```python
from build123d import *

# Parameters (mm, degrees)
SKETCH1_W                    = 39.4
SKETCH1_H                    = 49.4
BOSS_EXTRUDE1_DEPTH          = 1
SKETCH2_R                    = 7.25
CUT_EXTRUDE1_DEPTH           = 32.609808604
BOSS_EXTRUDE2_START          = -1
SKETCH3_R                    = 2.2
SKETCH3_R_2                  = 1
BOSS_EXTRUDE2_DEPTH          = 10.4
SKETCH4_W                    = 39.4
SKETCH4_H                    = 49.4
SKETCH4_W_2                  = 27.4
SKETCH4_H_2                  = 37.4
BOSS_EXTRUDE4_DEPTH          = 9.4
SKETCH5_W                    = 39.4
SKETCH5_H                    = 6
BOSS_EXTRUDE5_DEPTH          = 10
SKETCH6_R                    = 1.65
CUT_EXTRUDE3_DEPTH           = 57.961478211
SKETCH7_R                    = 2.25
CUT_EXTRUDE4_DEPTH           = 57.961478211
BOSS_EXTRUDE6_START          = -9.4
BOSS_EXTRUDE6_DEPTH          = 9.4
SKETCH9_R                    = 1.1
CUT_EXTRUDE5_DEPTH           = 8
CUT_EXTRUDE5_DRAFT           = -2
CUT_EXTRUDE5_PROFILE_2_DEPTH = 8
CUT_EXTRUDE5_PROFILE_2_DRAFT = -2
CUT_EXTRUDE5_PROFILE_3_DEPTH = 8
CUT_EXTRUDE5_PROFILE_3_DRAFT = -2
CUT_EXTRUDE5_PROFILE_4_DEPTH = 8
CUT_EXTRUDE5_PROFILE_4_DRAFT = -2
CHAMFER1_SIZE                = 5


with BuildPart() as part:
    # Sketch1 → Boss-Extrude1 (new body)
    with BuildSketch(Plane.XY):
        Rectangle(SKETCH1_W, SKETCH1_H)
    extrude(amount=BOSS_EXTRUDE1_DEPTH)

    # Sketch2 → Cut-Extrude1 (cut, through all)
    with BuildSketch(Plane.XY.offset(1)):
        Circle(SKETCH2_R)
    extrude(amount=-CUT_EXTRUDE1_DEPTH, mode=Mode.SUBTRACT)

    # Sketch3 → Boss-Extrude2 (add)
    # profile 1 of 4: a face of its own
    with BuildSketch(Plane.XY.offset(1).offset(BOSS_EXTRUDE2_START)):
        with Locations(Location((-10.5, 4.98, 0), (0, 0, 180))):
            Circle(SKETCH3_R)
        with Locations(Location((-10.5, 4.98, 0), (0, 0, 180))):
            Circle(SKETCH3_R_2, mode=Mode.SUBTRACT)
    # profile 2 of 4: a face of its own
    with BuildSketch(Plane.XY.offset(1).offset(BOSS_EXTRUDE2_START)):
        with Locations(Location((-10.5, -7.52, 0), (0, 0, 180))):
            Circle(SKETCH3_R)
        with Locations(Location((-10.5, -7.52, 0), (0, 0, 180))):
            Circle(SKETCH3_R_2, mode=Mode.SUBTRACT)
    # profile 3 of 4: a face of its own
    with BuildSketch(Plane.XY.offset(1).offset(BOSS_EXTRUDE2_START)):
        with Locations(Location((10.5, -7.52, 0), (0, 0, 180))):
            Circle(SKETCH3_R)
        with Locations(Location((10.5, -7.52, 0), (0, 0, 180))):
            Circle(SKETCH3_R_2, mode=Mode.SUBTRACT)
    # profile 4 of 4: a face of its own
    with BuildSketch(Plane.XY.offset(1).offset(BOSS_EXTRUDE2_START)):
        with Locations(Location((10.5, 4.98, 0), (0, 0, 180))):
            Circle(SKETCH3_R)
        with Locations(Location((10.5, 4.98, 0), (0, 0, 180))):
            Circle(SKETCH3_R_2, mode=Mode.SUBTRACT)
    extrude(amount=BOSS_EXTRUDE2_DEPTH)

    # Sketch4 → Boss-Extrude4 (add)
    with BuildSketch(Plane.XY.offset(1)):
        Rectangle(SKETCH4_W, SKETCH4_H)
        Rectangle(SKETCH4_W_2, SKETCH4_H_2, mode=Mode.SUBTRACT)
    extrude(amount=BOSS_EXTRUDE4_DEPTH)

    # Sketch5 → Boss-Extrude5 (add)
    with BuildSketch(Plane.XY.offset(10.4)):
        with Locations((0, 21.7)):
            Rectangle(SKETCH5_W, SKETCH5_H)
        with Locations((0, -21.7)):
            Rectangle(SKETCH5_W, SKETCH5_H)
    extrude(amount=BOSS_EXTRUDE5_DEPTH)

    # Sketch6 → Cut-Extrude3 (cut, through all)
    with BuildSketch(Plane(origin=(0, 24.7, 0), x_dir=(1, 0, 0), z_dir=(0, 1, 0))):
        with Locations(Location((-12.5, -12.4, 0), (0, 0, 180))):
            Circle(SKETCH6_R)
        with Locations(Location((12.5, -12.4, 0), (0, 0, 180))):
            Circle(SKETCH6_R)
    extrude(amount=-CUT_EXTRUDE3_DEPTH, mode=Mode.SUBTRACT)

    # Sketch7 → Cut-Extrude4 (cut, through all)
    with BuildSketch(Plane(origin=(0, 24.7, 0), x_dir=(1, 0, 0), z_dir=(0, 1, 0))):
        with Locations(Location((12.5, -12.4, 0), (0, 0, 180))):
            Circle(SKETCH7_R)
        with Locations(Location((-12.5, -12.4, 0), (0, 0, 180))):
            Circle(SKETCH7_R)
    extrude(amount=-CUT_EXTRUDE4_DEPTH, mode=Mode.SUBTRACT)

    # Sketch8 → Boss-Extrude6 (add)
    with BuildSketch(Plane.XY.offset(10.4).offset(BOSS_EXTRUDE6_START)):
        with BuildLine():
            Line((-10.5, 7.18), (-13.7, 7.18))
            Line((-13.7, 7.18), (-13.7, 2.78))
            Line((-13.7, 2.78), (-10.5, 2.78))
            ThreePointArc((-10.5, 2.78), (-8.3, 4.98), (-10.5, 7.18))
        make_face()
        with BuildLine():
            Line((-10.5, -5.32), (-13.7, -5.32))
            Line((-13.7, -5.32), (-13.7, -9.72))
            Line((-13.7, -9.72), (-10.5, -9.72))
            ThreePointArc((-10.5, -9.72), (-8.3, -7.52), (-10.5, -5.32))
        make_face()
        with BuildLine():
            Line((10.5, 7.18), (13.7, 7.18))
            Line((13.7, 7.18), (13.7, 2.78))
            Line((13.7, 2.78), (10.5, 2.78))
            ThreePointArc((10.5, 2.78), (8.3, 4.98), (10.5, 7.18))
        make_face()
        with BuildLine():
            Line((10.5, -5.32), (13.7, -5.32))
            Line((13.7, -5.32), (13.7, -9.72))
            Line((13.7, -9.72), (10.5, -9.72))
            ThreePointArc((10.5, -9.72), (8.3, -7.52), (10.5, -5.32))
        make_face()
    extrude(amount=BOSS_EXTRUDE6_DEPTH)


with BuildPart() as cut_extrude5_tool:
    # Sketch9 → Cut-Extrude5 (with draft: the straight prism first)
    with BuildSketch(Plane.XY.offset(10.4)):
        with Locations((-10.5, 4.98)):
            Circle(SKETCH9_R)
    extrude(amount=-CUT_EXTRUDE5_DEPTH)
    # Cut-Extrude5: the draft: its side faces are tilted about the plane it starts from
    cut_extrude5_sides = [cut_extrude5_tool.faces().sort_by_distance(p)[0] for p in [
        (-11.6, 4.98, 6.4),
    ]]
    draft(cut_extrude5_sides, Plane.XY.offset(10.4), CUT_EXTRUDE5_DRAFT)


with BuildPart() as part_1:
    add(part.part)

    # Cut-Extrude5: cut by cut_extrude5_tool
    add(cut_extrude5_tool.part, mode=Mode.SUBTRACT)


with BuildPart() as cut_extrude5_profile_2_tool:
    # Sketch9 → Cut-Extrude5 profile 2 (with draft: the straight prism first)
    with BuildSketch(Plane.XY.offset(10.4)):
        with Locations((10.5, 4.98)):
            Circle(SKETCH9_R)
    extrude(amount=-CUT_EXTRUDE5_PROFILE_2_DEPTH)
    # Cut-Extrude5 profile 2: the draft: its side faces are tilted about the plane it starts from
    cut_extrude5_profile_2_sides = [cut_extrude5_profile_2_tool.faces().sort_by_distance(p)[0] for p in [
        (9.4, 4.98, 6.4),
    ]]
    draft(cut_extrude5_profile_2_sides, Plane.XY.offset(10.4), CUT_EXTRUDE5_PROFILE_2_DRAFT)


with BuildPart() as part_2:
    add(part_1.part)

    # Cut-Extrude5 profile 2: cut by cut_extrude5_profile_2_tool
    add(cut_extrude5_profile_2_tool.part, mode=Mode.SUBTRACT)


with BuildPart() as cut_extrude5_profile_3_tool:
    # Sketch9 → Cut-Extrude5 profile 3 (with draft: the straight prism first)
    with BuildSketch(Plane.XY.offset(10.4)):
        with Locations((10.5, -7.52)):
            Circle(SKETCH9_R)
    extrude(amount=-CUT_EXTRUDE5_PROFILE_3_DEPTH)
    # Cut-Extrude5 profile 3: the draft: its side faces are tilted about the plane it starts from
    cut_extrude5_profile_3_sides = [cut_extrude5_profile_3_tool.faces().sort_by_distance(p)[0] for p in [
        (9.4, -7.52, 6.4),
    ]]
    draft(cut_extrude5_profile_3_sides, Plane.XY.offset(10.4), CUT_EXTRUDE5_PROFILE_3_DRAFT)


with BuildPart() as part_3:
    add(part_2.part)

    # Cut-Extrude5 profile 3: cut by cut_extrude5_profile_3_tool
    add(cut_extrude5_profile_3_tool.part, mode=Mode.SUBTRACT)


with BuildPart() as cut_extrude5_profile_4_tool:
    # Sketch9 → Cut-Extrude5 profile 4 (with draft: the straight prism first)
    with BuildSketch(Plane.XY.offset(10.4)):
        with Locations((-10.5, -7.52)):
            Circle(SKETCH9_R)
    extrude(amount=-CUT_EXTRUDE5_PROFILE_4_DEPTH)
    # Cut-Extrude5 profile 4: the draft: its side faces are tilted about the plane it starts from
    cut_extrude5_profile_4_sides = [cut_extrude5_profile_4_tool.faces().sort_by_distance(p)[0] for p in [
        (-11.6, -7.52, 6.4),
    ]]
    draft(cut_extrude5_profile_4_sides, Plane.XY.offset(10.4), CUT_EXTRUDE5_PROFILE_4_DRAFT)


with BuildPart() as part_4:
    add(part_3.part)

    # Cut-Extrude5 profile 4: cut by cut_extrude5_profile_4_tool
    add(cut_extrude5_profile_4_tool.part, mode=Mode.SUBTRACT)

    # Chamfer1
    chamfer1_edges = [part_4.edges().sort_by_distance(p)[0] for p in [
        (0, 24.7, 0),
        (0, -24.7, 0),
    ]]
    chamfer(chamfer1_edges, length=CHAMFER1_SIZE)


solid = part_4.part
```
Geometry check sheet. Reference: the model listing, model coordinates, mm. A direction names the side the tool comes from. Round coordinates to 2 decimals unless told otherwise and drop trailing zeros. Loops run counter-clockwise (first coordinate to the right, second up) from the corner with the lowest first, then second, coordinate; pieces in that order, holes last. Notation, with made-up numbers: M 38.25,-10.75 L 48.25,-10.75 A8 ccw 48.25,-1.75 Z; hole C -24.75,23.25 d5. An arc over 180 degrees is marked long. Return JSON: item names as keys, results as strings. Group by question number.
(1) Section check B-B, the plane x = 0. Enter the section's corners in (y, z).
(2) Section check D-D, the plane y = 0. Enter the section's corners in (x, z), and give its area (3 significant figures).
(3) Set-up check for faces 4 (the face through (16, 0, 10.4)), 5 (the face through (3.35, -6.43, 0.51)), 6 (the face through (-13.7, -1, 6)): record each of +Z, -Z, +X, -X, +Y, -Y from which the full face is reachable in a straight line by a thin tool's end or side.
(4) Section check A-A, the plane z = 16.75. Enter the section's corners in (x, y), and give its area (3 significant figures).
(5) Scan lines: line 1 along X through (y, z) = (12, 3); line 2 along Y through (x, z) = (4, 15.25); line 3 along Y through (x, z) = (11, 3.25). Record each from-to range of solid material in increasing order. Write a range as [from, to].
(6) Go/stop test with flat-tipped pins: pin 1 (3.5 mm diameter, centred on x = 15.5, y = -3.5, fed in from +Z); pin 2 (1.3 mm diameter, centred on x = -10.5, y = -7.5, fed in from +Z); pin 3 (8.5 mm diameter, centred on x = 0, y = 0, fed in from -Z); pin 4 (2 mm diameter, centred on x = -11.5, y = 9.5, fed in from +Z). Record where each tip stops, or that it passes through.
(7) Mould release check, pull along Y, two halves, no side actions. Record for faces 1 (the face through (10.5, -7.5, 2.4)), 2 (the face through (19.7, 0, 8)), 3 (the face through (0, -24.7, 13)): pulls with the +Y half, pulls with the -Y half, needs draft (parallel to the pull), parting line crosses it, or undercut.
(8) Section check C-C, the plane x = 12.5. Enter the section's corners in (y, z).
Data:
{
 "1": {"outline": "M -24.7,5 L -19.7,0 L -7.25,0 L -7.25,1 L -18.7,1 L -18.7,20.4 L -24.7,20.4 Z; M 7.25,0 L 19.7,0 L 24.7,5 L 24.7,20.4 L 18.7,20.4 L 18.7,1 L 7.25,1 Z"},
 "2": {"outline": "M -19.7,0 L -7.25,0 L -7.25,1 L -13.7,1 L -13.7,10.4 L -19.7,10.4 Z; M 7.25,0 L 19.7,0 L 19.7,10.4 L 13.7,10.4 L 13.7,1 L 7.25,1 Z", "area": "138 mm²"},
 "3": {"face 4": "+Z, +X, -X", "face 5": "+Z, -Z", "face 6": "+Z"},
 "4": {"outline": "M -19.7,-24.7 L 19.7,-24.7 L 19.7,-18.7 L -19.7,-18.7 Z; M -19.7,18.7 L 19.7,18.7 L 19.7,24.7 L -19.7,24.7 Z", "area": "473 mm²"},
 "5": {"line 1": "[-19.7, -13.7], [13.7, 19.7]", "line 2": "[-24.7, -18.7], [18.7, 24.7]", "line 3": "[-22.95, -18.7], [-9.72, -8.21], [-6.83, -5.32], [2.78, 4.29], [5.67, 7.18], [18.7, 22.95]"},
 "6": {"pin 1": "z = 10.4", "pin 2": "z = 2.4", "pin 3": "through", "pin 4": "z = 1"},
 "7": {"face 1": "undercut", "face 2": "needs draft", "face 3": "pulls with the -Y half"},
 "8": {"outline": "M -24.7,5 L -19.7,0 L 19.7,0 L 24.7,5 L 24.7,10.15 L 18.7,10.15 L 18.7,1 L 7.18,1 L 7.18,10.4 L 2.78,10.4 L 2.78,1 L -5.32,1 L -5.32,10.4 L -9.72,10.4 L -9.72,1 L -18.7,1 L -18.7,10.15 L -24.7,10.15 Z; M -24.7,14.65 L -18.7,14.65 L -18.7,20.4 L -24.7,20.4 Z; M 18.7,14.65 L 24.7,14.65 L 24.7,20.4 L 18.7,20.4 Z"}
}
